```python
from build123d import *

# Parameters (mm, degrees)
SKETCH1_R                 = 78.359
BOSS_EXTRUDE1_DEPTH       = 25.4
SKETCH6_R                 = 76.1746
BOSS_EXTRUDE5_DEPTH       = 9.525
SKETCH7_R                 = 76.1746
BOSS_EXTRUDE6_DEPTH       = 9.525
SKETCH8_R                 = 73.025
CUT_EXTRUDE5_DEPTH        = 34.925
CUT_EXTRUDE3_START        = 25.4
SKETCH1_7_R               = 78.359
SKETCH1_7_R_2             = 76.1746
CUT_EXTRUDE3_DEPTH        = 9.525
CIRPATTERN2_COUNT         = 3
SKETCH4_R                 = 73.025
BOSS_EXTRUDE4_DEPTH       = 9.525
SKETCH9_R                 = 3.3
CUT_EXTRUDE6_DEPTH        = 45.45
SKETCH10_R                = 82.322787435
CUT_EXTRUDE7_DEPTH        = 35.925
TAP_DRILL_FOR_4_40_TAP1_D = 2.2606
CUT_EXTRUDE9_DEPTH        = 10.525
CIRPATTERN3_COUNT         = 4


with BuildPart() as part:
    # Sketch1 → Boss-Extrude1 (new body)
    with BuildSketch(Plane(origin=(0, 0, 0), x_dir=(1, 0, 0), z_dir=(0, 1, 0))):
        Circle(SKETCH1_R)
    extrude(amount=BOSS_EXTRUDE1_DEPTH)

    # Sketch6 → Boss-Extrude5 (add)
    with BuildSketch(Plane(origin=(0, 25.4, 0), x_dir=(1, 0, 0), z_dir=(0, 1, 0))):
        Circle(SKETCH6_R)
    extrude(amount=BOSS_EXTRUDE5_DEPTH)

    # Sketch7 → Boss-Extrude6 (add)
    with BuildSketch(Plane.XZ):
        Circle(SKETCH7_R)
    extrude(amount=BOSS_EXTRUDE6_DEPTH)

    # Sketch8 → Cut-Extrude5 (cut)
    with BuildSketch(Plane.XZ.offset(9.525)):
        Circle(SKETCH8_R)
    extrude(amount=-CUT_EXTRUDE5_DEPTH, mode=Mode.SUBTRACT)

    # Sketch1_7 → Cut-Extrude3 (cut)
    with BuildSketch(Plane(origin=(0, 0, 0), x_dir=(1, 0, 0), z_dir=(0, 1, 0)).offset(CUT_EXTRUDE3_START)):
        Circle(SKETCH1_7_R)
        Circle(SKETCH1_7_R_2, mode=Mode.SUBTRACT)
    cut_extrude3 = extrude(amount=-CUT_EXTRUDE3_DEPTH, mode=Mode.SUBTRACT)

    # CirPattern2: Cut-Extrude3 ×3 about axis
    cirpattern2_axis = Axis((0, 0, 0), (0, 1, 0))
    for i in range(1, CIRPATTERN2_COUNT):
        add(cut_extrude3.rotate(cirpattern2_axis, i * 360 / CIRPATTERN2_COUNT), mode=Mode.SUBTRACT)

    # Sketch4 → Boss-Extrude4 (add)
    with BuildSketch(Plane(origin=(0, 34.925, 0), x_dir=(1, 0, 0), z_dir=(0, 1, 0))):
        Circle(SKETCH4_R)
    extrude(amount=-BOSS_EXTRUDE4_DEPTH)

    # Sketch9 → Cut-Extrude6 (cut, through all)
    with BuildSketch(Plane(origin=(0, 34.925, 0), x_dir=(1, 0, 0), z_dir=(0, 1, 0))):
        Circle(SKETCH9_R)
        with Locations((-19.546451191, -53.703433278)):
            Circle(SKETCH9_R)
        with Locations((-36.735311894, 43.779439924)):
            Circle(SKETCH9_R)
        with Locations((56.281763085, 9.923993354)):
            Circle(SKETCH9_R)
        with Locations((18.367655947, -21.889719962)):
            Circle(SKETCH9_R)
    extrude(amount=-CUT_EXTRUDE6_DEPTH, mode=Mode.SUBTRACT)

    # Sketch10 → Cut-Extrude7 (cut, through all)
    with BuildSketch(Plane(origin=(0, 25.4, 0), x_dir=(1, 0, 0), z_dir=(0, 1, 0))):
        Circle(SKETCH10_R)
    extrude(amount=-CUT_EXTRUDE7_DEPTH, mode=Mode.SUBTRACT)

    # Tap Drill for _4-40 Tap1 (through all)
    with Locations(Plane(origin=(0, 34.925, 0), x_dir=(1, 0, 0), z_dir=(0, 1, 0))):
        with Locations((7.384214894, 20.287963683), (15.934718491, 43.780279238)):
            Hole(TAP_DRILL_FOR_4_40_TAP1_D / 2)

    # Sketch14 → Cut-Extrude9 (cut, through all)
    with BuildSketch(Plane(origin=(0, 34.925, 0), x_dir=(1, 0, 0), z_dir=(0, 1, 0))):
        with BuildLine():
            Line((14.64382936, 22.781402035), (19.893154532, 37.203804415))
            ThreePointArc((19.893154532, 37.203804415), (19.808357055, 39.145985964), (18.37506644, 40.459354836))
            Line((18.37506644, 40.459354836), (11.930654446, 42.804928978))
            ThreePointArc((11.930654446, 42.804928978), (9.988472897, 42.720131501), (8.675104025, 41.286840886))
            Line((8.675104025, 41.286840886), (3.425778853, 26.864438506))
            ThreePointArc((3.425778853, 26.864438506), (3.51057633, 24.922256957), (4.943866945, 23.608888085))
            Line((4.943866945, 23.608888085), (11.388278939, 21.263313942))
            ThreePointArc((11.388278939, 21.263313942), (13.330460488, 21.34811142), (14.64382936, 22.781402035))
        make_face()
    extrude(amount=-CUT_EXTRUDE9_DEPTH, mode=Mode.SUBTRACT)

    # Sketch19 → Tap Drill for M4x0.7 Tap1 (revolve, cut)
    with BuildSketch(Plane(origin=(-38.0873, 30.1625, 65.969138723), x_dir=(0.866025404, 0, 0.5), z_dir=(0, 1, 0))):
        Polygon((0, 0), (0, 10.991425421), (1.65, 10.0000054), (1.65, 0.025), (1.675, 0), align=None)
    tap_drill_for_m4x0_7_tap1 = revolve(axis=Axis((-41.2623, 30.1625, 71.468400037), (0.5, 0, -0.866025404)), mode=Mode.SUBTRACT)

    # CirPattern3: Tap Drill for M4x0.7 Tap1 ×4 about axis
    cirpattern3_axis = Axis((0, 34.925, 0), (0, 1, 0))
    for i in range(1, CIRPATTERN3_COUNT):
        add(tap_drill_for_m4x0_7_tap1.rotate(cirpattern3_axis, i * 360 / CIRPATTERN3_COUNT), mode=Mode.SUBTRACT)


solid = part.part
```
Geometry: final body of the model. Coordinates: model frame, mm. A direction names the side the tool comes from. Round coordinates to 2 decimals unless told otherwise and drop trailing zeros. Write each loop counter-clockwise with the first axis right and the second up, starting at its lowest first coordinate (ties: lowest second). Pieces come first, ordered by that corner, then holes. Notation, with made-up numbers: M 71,19 L 106,19 A23 ccw 106,58 Z; hole C 43,22.25 d10. An arc over 180 degrees is marked long. Answer in a Markdown table with one row per item. Add a question column.
(1) Reachability of faces 1 (the face through (15.198, 30.229, -41.616)), 2 (the face through (-1, 25.4, 16)) from +Z, -Z, +X, -X, +Y, -Y: full face, straight path, thin tool, end or side. Return the list, or none.
(2) Cut plane A-A, the plane x = 0. Return the cut outline in (y, z) (3 decimals), then the cut area to 3 significant figures.
(3) Cut plane C-C, the plane z = 47. Return the cut outline in (x, y) (3 decimals).
(4) Cut plane B-B, the plane z = 0. Return the cut outline in (x, y) (3 decimals), then the cut area to 3 significant figures.
(5) Contact query for flat-ended pins moving along their axis: pin 1 (4 mm diameter, centred on x = -2.5, y = 27, fed in from +Z); pin 2 (4 mm diameter, centred on y = 33.5, z = -55.5, fed in from +X); pin 3 (3 mm diameter, centred on y = 31, z = 6, fed in from -X). Output: stop coordinate, or through.
(6) Ray query, L1, parallel to X at y = 32.25, z = 0; L2, parallel to X at y = 32.5, z = -43; L3, parallel to Z at x = -22.5, y = 27.5. Return the intervals inside material, ascending.
(7) Draft query along Z for faces 3 (the face through (3.5, 30.23, -24.95)), 4 (the face through (-16.513, 30.229, 74.363)), 5 (the face through (-1, 34.925, 16)). Return one class per face: pulls with the +Z half, pulls with the -Z half, needs draft (parallel to the pull), parting line crosses it, or undercut.
Established:
| question | item | result |
|---|---|---|
| 1 | face 1 | +Y, -Y |
| 1 | face 2 | +Z, -Z, +X, -X, -Y |
| 2 | outline | M 25.4,-76.175 L 34.925,-76.175 L 34.925,-3.3 L 25.4,-3.3 Z; M 25.4,3.3 L 34.925,3.3 L 34.925,76.175 L 25.4,76.175 Z |
| 2 | area | 1,390 mm² |
| 3 | outline | M -59.946,25.4 L 59.946,25.4 L 59.946,34.925 L -59.946,34.925 Z |
| 4 | outline | M -76.175,25.4 L -3.3,25.4 L -3.3,34.925 L -76.175,34.925 Z; M 3.3,25.4 L 76.175,25.4 L 76.175,34.925 L 3.3,34.925 Z |
| 4 | area | 1,390 mm² |
| 5 | pin 1 | z = 76.17 |
| 5 | pin 2 | x = 54.22 |
| 5 | pin 3 | x = -76.04 |
| 6 | L1 | -76.17 to -3.3, 3.3 to 76.17 |
| 6 | L2 | -62.88 to -39.94, -33.53 to 15.12, 16.75 to 62.88 |
| 6 | L3 | -72.78 to 52.23, 55.18 to 72.78 |
| 7 | face 3 | undercut |
| 7 | face 4 | parting line crosses it |
| 7 | face 5 | needs draft |
